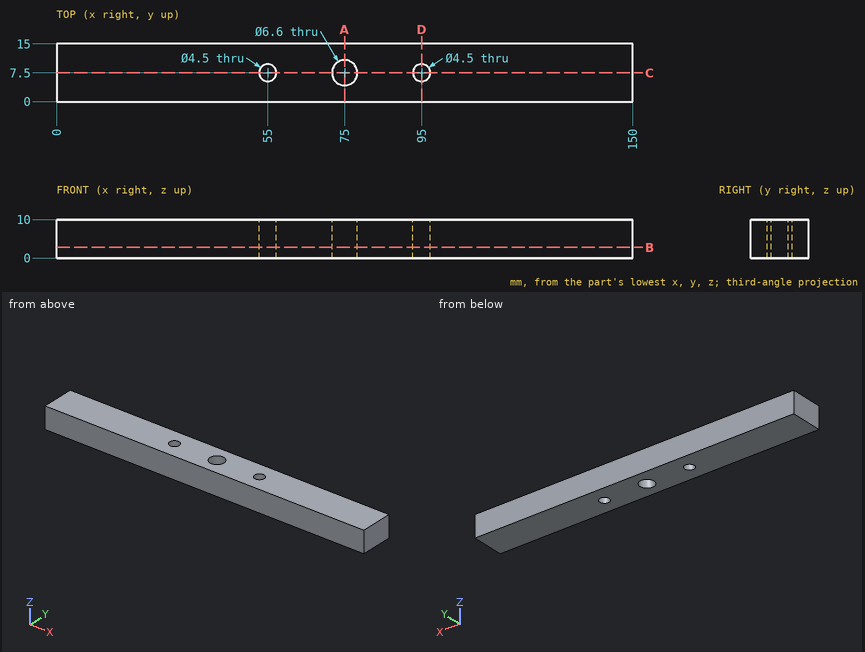
Part print with two shaded views. Sizes in mm from the minimum x, y, z corner. Coordinates: 2 decimals unless noted, no trailing zeros. Order: outer loops, then holes, each group sorted by start corner. A loop starts at its lowest first (then second) coordinate and runs counter-clockwise, first axis right, second up. Notation, with made-up numbers: M 67,87.25 L 81,87.25 A11 cw 81,108.25 Z; hole C 25,29 d4. An arc over 180 degrees is marked long. Use a Markdown table: item, result.
(1) Cut at B-B on z = 2.75. Write the cut outline in (x, y), then the cut area to 3 significant figures.
A:
| item | result |
|---|---|
| outline | M 0,0 L 150,0 L 150,15 L 0,15 Z; hole C 55,7.5 d4.5; hole C 75,7.5 d6.6; hole C 95,7.5 d4.5 |
| area | 2,180 mm^2 |
(2) Cut at C-C on y = 7.5. Write the cut outline in (x, z).
A:
| item | result |
|---|---|
| outline | M 0,0 L 52.75,0 L 52.75,10 L 0,10 Z; M 57.25,0 L 71.7,0 L 71.7,10 L 57.25,10 Z; M 78.3,0 L 92.75,0 L 92.75,10 L 78.3,10 Z; M 97.25,0 L 150,0 L 150,10 L 97.25,10 Z |
(3) Cut at A-A on x = 75. Write the cut outline in (y, z), then the cut area to 3 significant figures.
A:
| item | result |
|---|---|
| outline | M 0,0 L 4.2,0 L 4.2,10 L 0,10 Z; M 10.8,0 L 15,0 L 15,10 L 10.8,10 Z |
| area | 84.0 mm^2 |
(4) Cut at D-D on x = 95. Write the cut outline in (y, z), then the cut area to 3 significant figures.
A:
| item | result |
|---|---|
| outline | M 0,0 L 5.25,0 L 5.25,10 L 0,10 Z; M 9.75,0 L 15,0 L 15,10 L 9.75,10 Z |
| area | 105 mm^2 |
(5) Probe L1, parallel to X at y = 7.5, z = 5.5; L2, parallel to Y at x = 75, z = 4.75; L3, parallel to X at y = 8.5, z = 7.5. List the from-to ranges inside material, lowest first.
A:
| item | result |
|---|---|
| L1 | x = 0 to 52.75, 57.25 to 71.7, 78.3 to 92.75, 97.25 to 150 |
| L2 | y = 0 to 4.2, 10.8 to 15 |
| L3 | x = 0 to 52.98, 57.02 to 71.86, 78.14 to 92.98, 97.02 to 150 |
